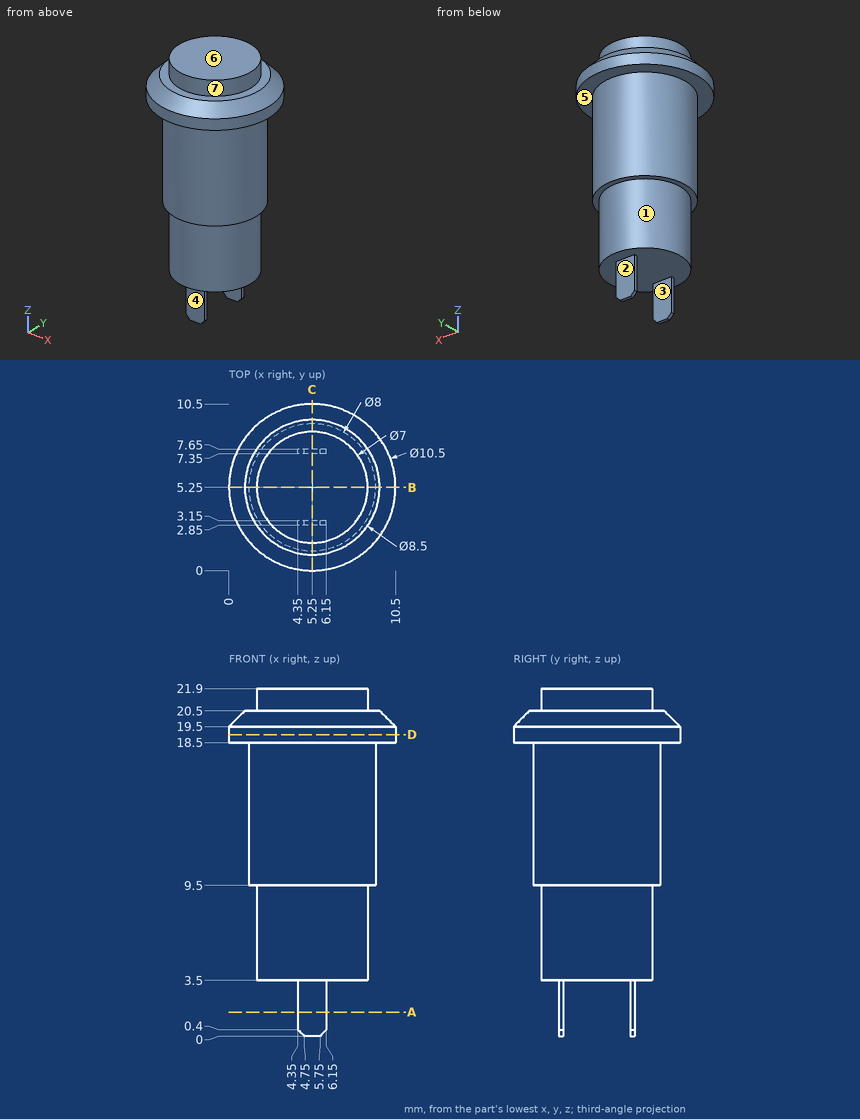
Design review of the part shown in the three views and the two pictorial views. Dimensions are in mm from the part's minimum x, y and z. A direction names the side the tool comes from. Round coordinates to 2 decimals unless told otherwise and drop trailing zeros. Write each loop counter-clockwise with the first axis right and the second up, starting at its lowest first coordinate (ties: lowest second). Pieces come first, ordered by that corner, then holes.
1) Take a section at A-A on z = 1.5. Give the boundary of the cut face in (x, y).
Answer below:
outline: (4.35, 2.85) - (6.15, 2.85) - (6.15, 3.15) - (4.35, 3.15) - close; (4.35, 7.35) - (6.15, 7.35) - (6.15, 7.65) - (4.35, 7.65) - close
2) Mouldability with a two-part tool opening along Y and no side actions: class the marked faces 1, 2 and 3 as +Y half, -Y half, draft (parallel to the pull), parting line (faces both ways), or undercut.
Answer below:
face 1: parting line
face 2: +Y half
face 3: undercut
3) Take a section at B-B on y = 5.25. Give the boundary of the cut face in (x, z).
Answer below:
outline: (0, 18.5) - (1.25, 18.5) - (1.25, 9.5) - (1.75, 9.5) - (1.75, 3.5) - (8.75, 3.5) - (8.75, 9.5) - (9.25, 9.5) - (9.25, 18.5) - (10.5, 18.5) - (10.5, 19.5) - (9.5, 20.5) - (8.75, 20.5) - (8.75, 21.9) - (1.75, 21.9) - (1.75, 20.5) - (1, 20.5) - (0, 19.5) - close
4) Take a section at C-C on x = 5.25. Give the boundary of the cut face in (y, z).
Answer below:
outline: (0, 18.5) - (1.25, 18.5) - (1.25, 9.5) - (1.75, 9.5) - (1.75, 3.5) - (2.85, 3.5) - (2.85, 0) - (3.15, 0) - (3.15, 3.5) - (7.35, 3.5) - (7.35, 0) - (7.65, 0) - (7.65, 3.5) - (8.75, 3.5) - (8.75, 9.5) - (9.25, 9.5) - (9.25, 18.5) - (10.5, 18.5) - (10.5, 19.5) - (9.5, 20.5) - (8.75, 20.5) - (8.75, 21.9) - (1.75, 21.9) - (1.75, 20.5) - (1, 20.5) - (0, 19.5) - close
5) Take a section at D-D on z = 19. Give the boundary of the cut face in (x, y).
Answer below:
outline: circle Ø10.5 at (5.25, 5.25)
6) Machinability: for the marked faces 4, 5, 6 and 7, which of the approach directions +Z, -Z, +X, -X, +Y, -Y give a long, thin tool a straight path to every point of the face, cutting with its end or side? Answer none if there is none.
Answer below:
face 4: -Z, +X, -X, -Y
face 5: -Z
face 6: +Z, +X, -X, +Y, -Y
face 7: +Z
7) For line 1 along Z through (x, y) = (9, 4); line 2 along Z through (x, y) = (5.5, 6.25); line 3 along X through (y, z) = (5.75, 17.75), list the stretches that pass through material, from the lowest coordinate up.
Answer below:
line 1: z = 9.5 to 20.5
line 2: z = 3.5 to 21.9
line 3: x = 1.28 to 9.22
8) Insertion check: pin 1 Ø3 at (x, y) = (1, 2) entering from +Z; pin 2 Ø1.4 at (x, z) = (5.5, 2) entering from +Y; pin 3 Ø1.5 at (x, z) = (1, 10.5) entering from -Y. Each pin has a flat end and moves straight along its axis. Give the tip position at first contact, or say it passes through.
Answer below:
pin 1: stops at z = 20.5
pin 2: stops at y = 7.65
pin 3: stops at y = 3.31
